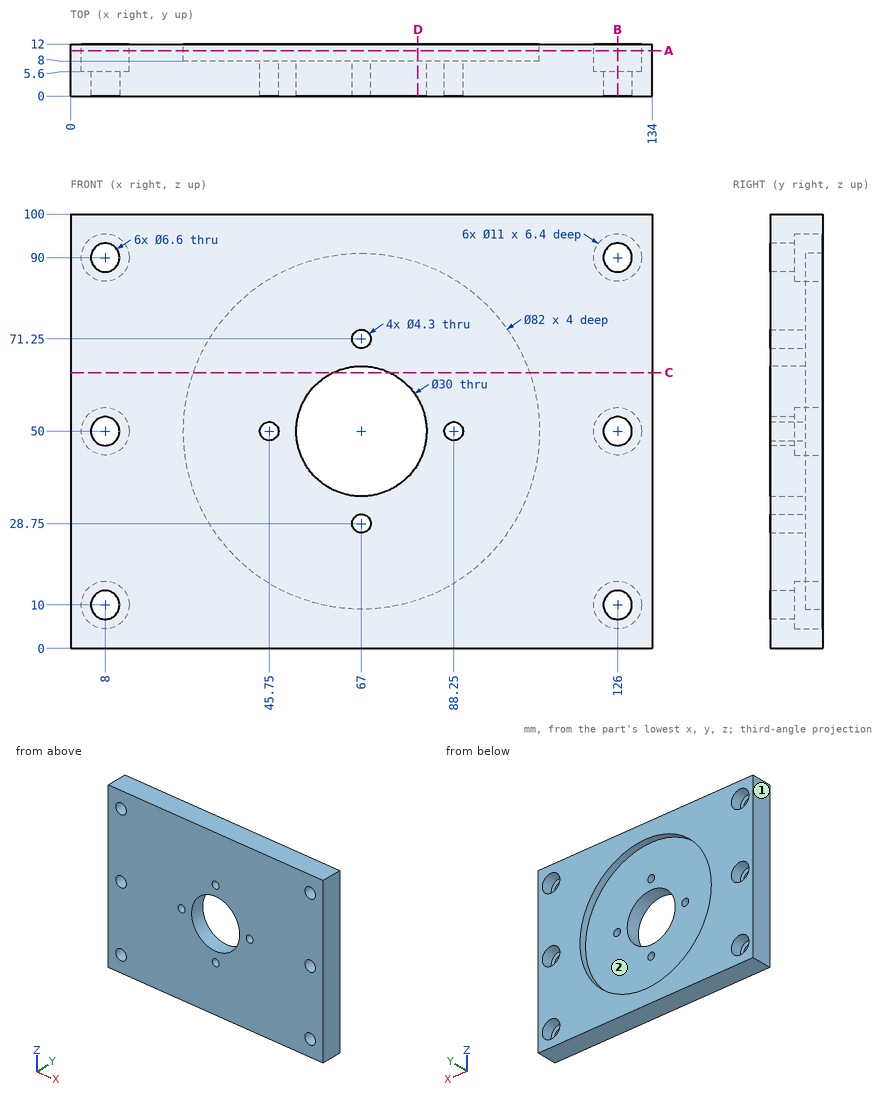
For this review, use the dimensioned drawing (mm, ordinates from the lowest corner) and the shaded views. Coordinates: 2 decimals unless noted, no trailing zeros. Loops run counter-clockwise (first coordinate to the right, second up) from the corner with the lowest first, then second, coordinate; pieces in that order, holes last. Notation, with made-up numbers: (5.25, 0.25) -> (51.25, 0.25) arc R20 cw to (51.25, 21.25) -> close; hole circle Ø6 at (35.5, -6). An arc over 180 degrees is marked (long way). Use a Markdown table: item, result. Add a question column.
Item 1: Wall thickness on L1, parallel to X at y = 2.3, z = 10; L2, parallel to X at y = 6.25, z = 50; L3, parallel to X at y = 9.55, z = 50: over which ranges is each line inside the solid? List them lowest first. Write a range as from..to.
Item 2: Clearance check with flat-ended pins moving along their axes: P1, Ø9, axis at x = 126, z = 50, coming from the +Y side; P2, Ø3.5, axis at x = 67, z = 28.75, coming from the +Y side; P3, Ø5, axis at x = 60, z = 26, coming from the +Y side. State where each tip first meets the part, or that it passes through.
Item 3: We need section C-C, the plane z = 63.5. Write out the cut boundary in (x, y).
Item 4: We need section A-A, the plane y = 10.5. Write out the cut boundary in (x, z).
Item 5: The part is to be moulded in two halves that separate along Z. For the marked faces 1 and 2, say which applies: +Z half, -Z half, draft (parallel to the pull), parting line (faces both ways), or undercut.
Item 6: We need section B-B, the plane x = 126. Write out the cut boundary in (y, z), and give its area (3 significant figures).
Item 7: We need section D-D, the plane x = 80. Write out the cut boundary in (y, z), and give its area (3 significant figures).
Numbers:
| question | item | result |
|---|---|---|
| 1 | L1 | x = 0..4.7, 11.3..122.7, 129.3..134 |
| 1 | L2 | x = 0..2.5, 13.5..43.6, 47.9..52, 82..86.1, 90.4..120.5, 131.5..134 |
| 1 | L3 | x = 0..2.5, 13.5..26, 108..120.5, 131.5..134 |
| 2 | P1 | stops at y = 5.6 |
| 2 | P2 | passes through |
| 2 | P3 | stops at y = 8 |
| 3 | outline | (0, 0) -> (60.46, 0) -> (60.46, 8) -> (28.29, 8) -> (28.29, 12) -> (0, 12) -> close; (73.54, 0) -> (134, 0) -> (134, 12) -> (105.71, 12) -> (105.71, 8) -> (73.54, 8) -> close |
| 4 | outline | (0, 0) -> (134, 0) -> (134, 100) -> (0, 100) -> close; hole circle Ø11 at (8, 10); hole circle Ø11 at (8, 50); hole circle Ø11 at (8, 90); hole circle Ø82 at (67, 50); hole circle Ø11 at (126, 10); hole circle Ø11 at (126, 50); hole circle Ø11 at (126, 90) |
| 5 | face 1 | draft |
| 5 | face 2 | undercut |
| 6 | outline | (0, 0) -> (12, 0) -> (12, 4.5) -> (5.6, 4.5) -> (5.6, 6.7) -> (0, 6.7) -> close; (0, 13.3) -> (5.6, 13.3) -> (5.6, 15.5) -> (12, 15.5) -> (12, 44.5) -> (5.6, 44.5) -> (5.6, 46.7) -> (0, 46.7) -> close; (0, 53.3) -> (5.6, 53.3) -> (5.6, 55.5) -> (12, 55.5) -> (12, 84.5) -> (5.6, 84.5) -> (5.6, 86.7) -> (0, 86.7) -> close; (0, 93.3) -> (5.6, 93.3) -> (5.6, 95.5) -> (12, 95.5) -> (12, 100) -> (0, 100) -> close |
| 6 | area | 878 mm^2 |
| 7 | outline | (0, 0) -> (12, 0) -> (12, 11.12) -> (8, 11.12) -> (8, 42.52) -> (0, 42.52) -> close; (0, 57.48) -> (8, 57.48) -> (8, 88.88) -> (12, 88.88) -> (12, 100) -> (0, 100) -> close |
| 7 | area | 769 mm^2 |
